```python
from build123d import *

# Parameters (mm, degrees)
F0_W     = 80
F0_H     = 80
F0_R     = 2.1
F0_R_2   = 4
F0_R_3   = 15
F0_R_4   = 6
F1_DEPTH = 10
F2_R     = 2.5
F3_DEPTH = 25
F4_R     = 3
F5_DEPTH = 4
F7_DEPTH = 5


with BuildPart() as f1:
    # F0 (on Top) → F1 (new body)
    with BuildSketch(Plane.XY):
        with Locations((40, -40)):
            Rectangle(F0_W, F0_H)
        with Locations((40.5, -54.699928)):
            Circle(F0_R, mode=Mode.SUBTRACT)
        with Locations((71.5, -54.699928)):
            Circle(F0_R, mode=Mode.SUBTRACT)
        with Locations((13, -11.199928)):
            Circle(F0_R_2, mode=Mode.SUBTRACT)
        with Locations((56, -39.199928)):
            Circle(F0_R_3, mode=Mode.SUBTRACT)
        with Locations((40.5, -23.699928)):
            Circle(F0_R, mode=Mode.SUBTRACT)
        with Locations((71.5, -23.699928)):
            Circle(F0_R, mode=Mode.SUBTRACT)
        with Locations((68, -11.199928)):
            Circle(F0_R_4, mode=Mode.SUBTRACT)
    extrude(amount=F1_DEPTH)

    # F2 (on face) → F3 (cut)
    with BuildSketch(Plane.XY.offset(10)):
        with Locations((26, -39.199928)):
            Circle(F2_R)
        with Locations((16, -69.349928)):
            Circle(F2_R)
        with Locations((66, -69.349928)):
            Circle(F2_R)
    extrude(amount=-F3_DEPTH, mode=Mode.SUBTRACT)

    # F4 (on face) → F5 (cut)
    with BuildSketch(Plane.XY.offset(10)):
        with Locations((40.5, -23.699928)):
            Circle(F4_R)
        with Locations((71.5, -23.699928)):
            Circle(F4_R)
        with Locations((40.5, -54.699928)):
            Circle(F4_R)
        with Locations((71.5, -54.699928)):
            Circle(F4_R)
    extrude(amount=-F5_DEPTH, mode=Mode.SUBTRACT)

    # F6 (on face) → F7 (cut)
    with BuildSketch(Plane.XY.offset(10)):
        Polygon((16.752777, -4.699928), (9.247223, -4.699928), (5.494447, -11.199928), (9.247223, -17.699928), (16.752777, -17.699928), (20.505553, -11.199928), align=None)
    extrude(amount=-F7_DEPTH, mode=Mode.SUBTRACT)


solid = f1.part
```
Work out the finished part from the listing and answer in its coordinate system (mm). A direction names the side the tool comes from. Round coordinates to 2 decimals unless told otherwise and drop trailing zeros. Write each loop counter-clockwise with the first axis right and the second up, starting at its lowest first coordinate (ties: lowest second). Pieces come first, ordered by that corner, then holes.
1) Determine the mould class of faces 1 (the face through (39, 0, 5)), 2 (the face through (71.04, -56.75, 2.96)), 3 (the face through (39, -39, 10)) for opening direction Y: pulls with the +Y half, pulls with the -Y half, needs draft (parallel to the pull), parting line crosses it, or undercut.
2) Which of the six approach directions +Z, -Z, +X, -X, +Y, -Y give full straight-line access (tool end or side, diameter ignored) to faces 4 (the face through (69.1, -25.5, 8)), 5 (the face through (65.67, -66.87, 5.07))?
3) A cutting plane is placed at C-C on x = 56. Determine the outline of the cut face in (y, z).
4) Consider probe 1 along Y at (x, z) = (40.5, 7.75); probe 2 along X at (y, z) = (-24, 2.5); probe 3 along Y at (x, z) = (40.5, 2.25). Determine where each line is inside the solid, lowest interval first.
5) A cutting plane is placed at B-B on x = 66. Determine the outline of the cut face in (y, z).
6) A cutting plane is placed at A-A on x = 10.5. Determine the outline of the cut face in (y, z).
Entries:
1. face 1: pulls with the +Y half
1. face 2: undercut
1. face 3: needs draft
2. face 4: +Z
2. face 5: +Z, -Z
3. outline: (-80, 0) - (-54.2, 0) - (-54.2, 10) - (-80, 10) - close; (-24.2, 0) - (0, 0) - (0, 10) - (-24.2, 10) - close
4. probe 1: y = -80 to -57.7, -51.7 to -26.7, -20.7 to 0
4. probe 2: x = 0 to 38.42, 42.58 to 69.42, 73.58 to 80
4. probe 3: y = -80 to -56.8, -52.6 to -25.8, -21.6 to 0
5. outline: (-80, 0) - (-71.85, 0) - (-71.85, 10) - (-80, 10) - close; (-66.85, 0) - (-50.38, 0) - (-50.38, 10) - (-66.85, 10) - close; (-28.02, 0) - (-16.86, 0) - (-16.86, 10) - (-28.02, 10) - close; (-5.54, 0) - (0, 0) - (0, 10) - (-5.54, 10) - close
6. outline: (-80, 0) - (-14.32, 0) - (-14.32, 5) - (-17.7, 5) - (-17.7, 10) - (-80, 10) - close; (-8.08, 0) - (0, 0) - (0, 10) - (-4.7, 10) - (-4.7, 5) - (-8.08, 5) - close
